Could you check a few things on this model? Use its own coordinates, in mm. A direction names the side the tool comes from. Coordinates: 2 decimals unless noted, no trailing zeros. Order: outer loops, then holes, each group sorted by start corner. A loop starts at its lowest first (then second) coordinate and runs counter-clockwise, first axis right, second up. Notation, with made-up numbers: (8.25, 68.25) - (21.25, 68.25) arc R24 ccw to (21.25, 80.25) - close; hole circle Ø9 at (73.5, 36). An arc over 180 degrees is marked (long way). One line per item, written item: value.
from build123d import *

# Parameters (mm, degrees)
SKETCH1_W                    = 50
SKETCH1_H                    = 50
BASE_FLANGE1_DEPTH           = 2.5
EDGE_FLANGE2_STRIP_W         = 21
EDGE_FLANGE2_STRIP_H         = 2.5
EDGE_FLANGE2_STRIP_CUT_DEPTH = 50
EDGE_FLANGE2_DEPTH           = 50
BREAK_CORNER2_START          = -25
BREAK_CORNER2_DEPTH          = 2.5
EDGE_FLANGE4_DEPTH           = 30
SKETCH29_R                   = 15
CUT_EXTRUDE1_DEPTH           = 10
CUT_EXTRUDE2_DEPTH           = 10
BREAK_CORNER3_START          = -30
BREAK_CORNER3_DEPTH          = 60
SKETCH31_R                   = 7.5
CUT_EXTRUDE3_DEPTH           = 72


# Read off the part's stored shape, not the designer's step: Break-Corner2, Break-Corner3
# Sheet-metal steps are written as plain solids
with BuildPart() as part:
    # Sketch1 → Base-Flange1 (new body)
    with BuildSketch(Plane(origin=(0, 0, 0), x_dir=(1, 0, 0), z_dir=(0, 1, 0))):
        Rectangle(SKETCH1_W, SKETCH1_H)
    extrude(amount=BASE_FLANGE1_DEPTH)

    # Edge-Flange2 strip (across the edge) → Edge-Flange2 strip cut (cut)
    with BuildSketch(Plane(origin=(25, 2.5, -25), x_dir=(0, 0, 1), z_dir=(-1, 0, 0))):
        with Locations((-2.5, -1.25)):
            Rectangle(EDGE_FLANGE2_STRIP_W, EDGE_FLANGE2_STRIP_H)
    extrude(amount=EDGE_FLANGE2_STRIP_CUT_DEPTH, mode=Mode.SUBTRACT)

    # Edge-Flange2 section (across the edge) → Edge-Flange2 (add)
    with BuildSketch(Plane(origin=(25, 2.5, -25), x_dir=(0, 0, 1), z_dir=(-1, 0, 0))):
        with BuildLine():
            Line((0, 5.5), (0, 57.5))
            Line((0, 57.5), (2.5, 57.5))
            Line((2.5, 57.5), (2.5, 5.5))
            ThreePointArc((2.5, 5.5), (4.110912703, 1.610912703), (8, 0))
            Line((8, 0), (8, -2.5))
            ThreePointArc((8, -2.5), (2.343145751, -0.156854249), (0, 5.5))
        make_face()
    extrude(amount=EDGE_FLANGE2_DEPTH)

    # Break-Corner2 outline → Break-Corner2 (cut)
    with BuildSketch(Plane.XY.offset(BREAK_CORNER2_START)):
        with BuildLine():
            ThreePointArc((-25, 35), (-17.67766953, 52.67766953), (0, 60))
            Line((0, 60), (-25, 60))
            Line((-25, 60), (-25, 35))
        make_face()
        with BuildLine():
            ThreePointArc((0, 60), (17.67766953, 52.67766953), (25, 35))
            Line((25, 35), (25, 60))
            Line((25, 60), (0, 60))
        make_face()
    extrude(amount=BREAK_CORNER2_DEPTH, mode=Mode.SUBTRACT)

    # Edge-Flange4 section (across the edge) → Edge-Flange4 (add)
    with BuildSketch(Plane(origin=(27.5, 2.5, 25), x_dir=(-1, 0, 0), z_dir=(0, 0, -1))):
        with BuildLine():
            Line((-2.5, 2.5), (-2.5, 37.5))
            Line((-2.5, 37.5), (0, 37.5))
            Line((0, 37.5), (0, 2.5))
            ThreePointArc((0, 2.5), (0.732233047, 0.732233047), (2.5, 0))
            Line((2.5, 0), (2.5, -2.5))
            ThreePointArc((2.5, -2.5), (-1.035533906, -1.035533906), (-2.5, 2.5))
        make_face()
    edge_flange4 = extrude(amount=EDGE_FLANGE4_DEPTH)

    # Mirror1: Edge-Flange4 across plane
    add(edge_flange4.mirror(Plane(origin=(0, 0, 0), x_dir=(0, 0, 1), z_dir=(1, 0, 0))))

    # Sketch29 → Cut-Extrude1 (cut)
    with BuildSketch(Plane.XY.offset(-22.5)):
        with Locations((0, 35)):
            Circle(SKETCH29_R)
    extrude(amount=-CUT_EXTRUDE1_DEPTH, mode=Mode.SUBTRACT)

    # Sketch30 → Cut-Extrude2 (cut)
    with BuildSketch(Plane(origin=(0, 2.5, 0), x_dir=(1, 0, 0), z_dir=(0, 1, 0))):
        with BuildLine():
            Line((-10, -43), (10, -43))
            Line((10, -43), (10, -7))
            ThreePointArc((10, -7), (0, 3), (-10, -7))
            Line((-10, -7), (-10, -43))
        make_face()
    extrude(amount=-CUT_EXTRUDE2_DEPTH, mode=Mode.SUBTRACT)

    # Break-Corner3 outline → Break-Corner3 (cut)
    with BuildSketch(Plane.YZ.offset(BREAK_CORNER3_START)):
        with BuildLine():
            Line((40, -5), (40, 10))
            ThreePointArc((40, 10), (35.606601718, -0.606601718), (25, -5))
            Line((25, -5), (40, -5))
        make_face()
        with BuildLine():
            ThreePointArc((25, 25), (35.606601718, 20.606601718), (40, 10))
            Line((40, 10), (40, 25))
            Line((40, 25), (25, 25))
        make_face()
    extrude(amount=BREAK_CORNER3_DEPTH, mode=Mode.SUBTRACT)

    # Sketch31 → Cut-Extrude3 (cut)
    with BuildSketch(Plane(origin=(30, 0, 0), x_dir=(0, 0, -1), z_dir=(1, 0, 0))):
        with Locations(Location((-10, 25, 0), (0, 0, 90))):
            Circle(SKETCH31_R)
    extrude(amount=-CUT_EXTRUDE3_DEPTH, mode=Mode.SUBTRACT)


solid = part.part
Item 1: I want a section at D-D on x = 22.5. Please give me the cut outline in (y, z).
Conclusion:
outline: (0, -17) arc R8 ccw to (8, -25) - (45.9, -25) - (45.9, -22.5) - (8, -22.5) arc R5.5 cw to (2.5, -17) - (2.5, 25) - (0, 25) - close
Item 2: I want a section at B-B on y = 37.5. Please give me the cut outline in (x, z), then the cut area to 3 significant figures.
Conclusion:
outline: (-30, 1.71) - (-27.5, 1.71) - (-27.5, 18.29) - (-30, 18.29) - close; (-24.87, -25) - (-14.79, -25) - (-14.79, -22.5) - (-24.87, -22.5) - close; (14.79, -25) - (24.87, -25) - (24.87, -22.5) - (14.79, -22.5) - close; (27.5, 1.71) - (30, 1.71) - (30, 18.29) - (27.5, 18.29) - close
area: 133 mm²
Item 3: Thinking about a two-plate mould opening in Y: for faces 4 (the face through (28.768, 19.048, 5.436)), 5 (the face through (-26.787, 3.252, 10.21)), 6 (the face through (-28.732, 19.048, 5.436)), 7 (the face through (0, 1, -3)), which applies, pulls with the +Y half, pulls with the -Y half, needs draft (parallel to the pull), parting line crosses it, or undercut?
Conclusion:
face 4: undercut
face 5: pulls with the +Y half
face 6: undercut
face 7: needs draft
Item 4: I want a section at A-A on x = -12. Please give me the cut outline in (y, z).
Conclusion:
outline: (0, -17) arc R8 ccw to (8, -25) - (26, -25) - (26, -22.5) - (8, -22.5) arc R5.5 cw to (2.5, -17) - (2.5, 25) - (0, 25) - close; (44, -25) - (56.93, -25) - (56.93, -22.5) - (44, -22.5) - close
Item 5: For faces 1 (the face through (-25, 12, -23)), 2 (the face through (26.787, 3.252, 10.21)), 3 (the face through (10, 1, 16)), which set-ups out of +Z, -Z, +X, -X, +Y, -Y let a thin tool reach every point of the face, with its end or its side?
Conclusion:
face 1: -Z, -X, +Y, -Y
face 2: +Z, -Z, +Y
face 3: +Z, +Y, -Y
Item 6: If I drill on probe 1 along X at (y, z) = (11, 7.5); probe 2 along Z at (x, y) = (-28, 25); probe 3 along Z at (x, y) = (4.5, 12), over which ranges is the centre line in solid material (lowest first)?
Conclusion:
probe 1: -30 to -27.5, 27.5 to 30
probe 2: -5 to 2.5, 17.5 to 25
probe 3: -25 to -22.5
Item 7: I want a section at C-C on z = 4. Please give me the cut outline in (x, y), then the cut area to 3 significant figures.
Conclusion:
outline: (-30, 5) arc R5 ccw to (-25, 0) - (-9.54, 0) - (-9.54, 2.5) - (-25, 2.5) arc R2.5 cw to (-27.5, 5) - (-27.5, 20.5) - (-30, 20.5) - close; (-30, 29.5) - (-27.5, 29.5) - (-27.5, 38.75) - (-30, 38.75) - close; (9.54, 0) - (25, 0) arc R5 ccw to (30, 5) - (30, 20.5) - (27.5, 20.5) - (27.5, 5) arc R2.5 cw to (25, 2.5) - (9.54, 2.5) - close; (27.5, 29.5) - (30, 29.5) - (30, 38.75) - (27.5, 38.75) - close
area: 230 mm²
Item 8: I'm going to push flat-ended pins straight in: pin 1 Ø2 at (y, z) = (1, 17.5) entering from -X; pin 2 Ø1.5 at (x, y) = (8, 18) entering from +Z; pin 3 Ø3 at (y, z) = (1, 17.5) entering from +X. Where does each tip first touch, or does it pass through?
Conclusion:
pin 1: x = -29
pin 2: z = -22.5
pin 3: x = 29.33
